Autodesk Fusion 360 part; units mm, degrees
sketch "Sketch1" plane through (0, 0, 0) normal (0, 1, 0) x (1, 0, 0) in component "2004745"
  line L0 (-11.1431, -112.4766) -> (81.2494, -112.4766) construction
  line L1 (-9.4032, -1.7834) -> (86.6433, -1.7834) construction
  line L2 (1.7327, -120.1324) -> (1.7327, 13.1495) construction
  line L3 (66.2487, -119.4365) -> (66.2487, -6.4824) construction
  line L4 (6.4317, -112.4766) -> (61.5497, -112.4766)
  line L5 (66.2487, -107.7776) -> (66.2487, -1.7834)
  line L6 (61.5497, -1.7834) -> (6.4317, -1.7834)
  line L7 (1.7327, -6.4824) -> (1.7327, -107.7776)
  arc A0 (6.4317, -1.7834) -> (1.7327, -6.4824) centre (6.4317, -6.4824) ccw
  arc A1 (66.2487, -6.4824) -> (61.5497, -1.7834) centre (61.5497, -6.4824) ccw
  arc A2 (1.7327, -107.7776) -> (6.4317, -112.4766) centre (6.4317, -107.7776) ccw
  arc A3 (61.5497, -112.4766) -> (66.2487, -107.7776) centre (61.5497, -107.7776) ccw
  line L8 (61.3465, -5.3394) -> (-4.4719, -5.3394) construction
  line L9 (76.7415, -108.9206) -> (-6.2738, -108.9206) construction
  line L10 (4.0949, 11.0388) -> (4.0949, -121.0301) construction
  line L11 (63.8865, 2.5767) -> (63.8865, -121.3323) construction
  line L12 (6.6349, -108.9206) -> (61.3465, -108.9206)
  line L13 (63.8865, -106.3806) -> (63.8865, -7.8794)
  line L14 (63.8865, -5.3394) -> (6.6349, -5.3394)
  line L15 (4.0949, -7.8794) -> (4.0949, -106.3806)
  arc A4 (4.0949, -106.3806) -> (6.6349, -108.9206) centre (6.6349, -106.3806) ccw
  arc A5 (61.3465, -108.9206) -> (63.8865, -106.3806) centre (61.3465, -106.3806) ccw
  arc A6 (6.6349, -5.3394) -> (4.0949, -7.8794) centre (6.6349, -7.8794) ccw
  arc A7 (63.8865, -7.8794) -> (61.3465, -5.3394) centre (61.3465, -7.8794) ccw
  dimension "d1" = 110.6932
  dimension "d2" = 64.516
  dimension "d3" = 4.699
  dimension "d4" = 4.699
  dimension "d5" = 4.699
  dimension "d6" = 4.699
  dimension "d7" = 3.556
  dimension "d8" = 3.556
  dimension "d9" = 2.3622
  dimension "d10" = 2.3622
  dimension "d11" = 2.54
  dimension "d12" = 2.54
  dimension "d13" = 2.54
  dimension "d14" = 2.54
extrude "Extrude1" add sketch "Sketch1" along normal blind 0.635 contours L12 L13 L14 L15 A4 A5 A6 A7 in component "2004745"
extrude "Extrude2" add sketch "Sketch1" against normal blind 2.7686 contours L4 L5 L6 L7 A0 A1 A2 A3 | L12 L13 L14 L15 A4 A5 A6 A7 in component "2004745"
chamfer "Chamfer1" distance 2.159 angle 45 8 edges at (33.9907, -2.7686, 1.7834) (64.8723, -2.7686, 3.1597) (66.2487, -2.7686, 57.13) (64.8723, -2.7686, 111.1003) (33.9907, -2.7686, 112.4766) (3.109, -2.7686, 111.1003) (1.7327, -2.7686, 57.13) (3.109, -2.7686, 3.1597) in component "2004745"
component "2004745" placed x (1, 0, 0) y (0, 1, 0) z (0, 0, 1) at (0, 0, 0)
equation "d17 = -0.134 in + 0.025 in"
For this review, take the finished solid that the model builds, in its own axes (mm). A direction names the side the tool comes from. Round coordinates to 2 decimals unless told otherwise and drop trailing zeros. Write each loop counter-clockwise with the first axis right and the second up, starting at its lowest first coordinate (ties: lowest second). Pieces come first, ordered by that corner, then holes. Notation, with made-up numbers: (22.25, -7.75) -> (51.25, -7.75) arc R20 ccw to (51.25, -0.75) -> close; hole circle Ø11 at (-37, -10.5). An arc over 180 degrees is marked (long way). One line per question, with ' | ' between items. Start each with the question number.
(1) Add section A-A, the plane z = 28. Write out the cut boundary in (x, y) (1 decimal), plus the area to 3 significant figures.
(2) Tool access review of faces 4 (the face through (4.86, 0.31, 108.2)), 5 (the face through (63.12, 0.31, 6.06)), 6 (the face through (64, -2, 110)), 7 (the face through (63.16, 0.31, 108.16)): name each direction out of +Z, -Z, +X, -X, +Y, -Y from which nothing blocks a thin tool from reaching the whole face with its end or side.
(3) Insertion check: P1, Ø0.7, axis at y = 0.5, z = 69, coming from the +X side. The pin has a flat end and moves straight along its axis. Give the tip position at first contact, or say it passes through.
(4) Add section C-C, the plane y = -1.9. Write out the cut boundary in (x, z), plus the area to 3 significant figures.
(5) Mouldability with a two-part tool opening along Y and no side actions: class faces 1 (the face through (4.82, 0.31, 6.1)), 2 (the face through (4.058, -1.914, 4.056)), 3 (the face through (3, 0, 57)) as released by +Y, released by -Y, zero draft, split by the parting line, or undercut.
(6) For line 1 along X through (y, z) = (0.3, 70); line 2 along Z through (x, y) = (56, 0.35); line 3 along X through (y, z) = (-2.45, 12), list the stretches that pass through material, from the lowest coordinate up. Write a range as from..to.
(7) Add section B-B, the plane x = 58. Write out the cut boundary in (y, z) (3 decimals).
Answer list:
1) outline: (1.7, -0.6) -> (3.9, -2.8) -> (64.1, -2.8) -> (66.2, -0.6) -> (66.2, 0) -> (63.9, 0) -> (63.9, 0.6) -> (4.1, 0.6) -> (4.1, 0) -> (1.7, 0) -> close | area: 212 mm²
2) face 4: +Z, -X, +Y | face 5: -Z, +X, +Y | face 6: +Z, +X, -Y | face 7: +Z, +X, +Y
3) P1: x = 63.89
4) outline: (3.02, 6.48) arc R3.41 ccw to (6.43, 3.07) -> (61.55, 3.07) arc R3.41 ccw to (64.96, 6.48) -> (64.96, 107.78) arc R3.41 ccw to (61.55, 111.19) -> (6.43, 111.19) arc R3.41 ccw to (3.02, 107.78) -> close | area: 6,690 mm²
5) face 1: zero draft | face 2: released by -Y | face 3: released by +Y
6) line 1: 4.09..63.89 | line 2: 5.34..108.92 | line 3: 3.57..64.41
7) outline: (-2.769, 3.942) -> (-0.61, 1.783) -> (0, 1.783) -> (0, 5.339) -> (0.635, 5.339) -> (0.635, 108.921) -> (0, 108.921) -> (0, 112.477) -> (-0.61, 112.477) -> (-2.769, 110.318) -> close
